The listing builds one solid part. Answer for the finished solid, in the listing's coordinates (mm). Round coordinates to 2 decimals unless told otherwise and drop trailing zeros. Order: outer loops, then holes, each group sorted by start corner. A loop starts at its lowest first (then second) coordinate and runs counter-clockwise, first axis right, second up. Notation, with made-up numbers: M 9,35.5 L 46,35.5 A21 cw 46,48.5 Z; hole C -11.75,-29 d5. An arc over 180 degrees is marked long. Put each result on its own line as item: value. Start each with the question number.
1. Consider line 1 (Y direction, x = 11.5, z = 546.1); line 2 (X direction, y = 8.25, z = 552). Determine where each line is inside the solid, lowest interval first.
2. The part is cut by section B-B (z = 322.5). Give the vertices of the cut face in (x, y), then the cut area to 3 significant figures.
3. The part is cut by section A-A (x = -5). Give the vertices of the cut face in (y, z), then the cut area to 3 significant figures.
Autodesk Inventor part; units mm, degrees
ref_plane "YZ Plane" through (0, 0, 0) normal (1, 0, 0) x (0, 1, 0)
ref_plane "XZ Plane" through (0, 0, 0) normal (0, 1, 0) x (-1, 0, 0)
ref_plane "XY Plane" through (0, 0, 0) normal (0, 0, 1) x (1, 0, 0)
sketch "Sketch1" plane through (0, 0, 0) normal (0, 0, 1) x (1, 0, 0)
  line L0 (-12.7, -12.7) -> (-12.7, 12.7)
  line L1 (-12.7, 12.7) -> (12.7, 12.7)
  line L2 (12.7, 12.7) -> (12.7, -12.7)
  line L3 (12.7, -12.7) -> (-12.7, -12.7)
  line L4 (-12.7, -12.7) -> (12.7, 12.7) construction
  line L5 (-12.7, 12.7) -> (12.7, -12.7) construction
  line L6 (11.1125, 11.1125) -> (-11.1125, 11.1125)
  line L7 (-11.1125, 11.1125) -> (-11.1125, -11.1125)
  line L8 (-11.1125, -11.1125) -> (11.1125, -11.1125)
  line L9 (11.1125, -11.1125) -> (11.1125, 11.1125)
  point P0 (0, 0)
  dimension "d0" = 25.4
  dimension "d1" = 25.4
  dimension "d2" = 1.5875
extrude "Extrusion1" add sketch "Sketch1" along normal blind 609.6
sketch "Sketch2" plane through (12.7, -12.7, 0) normal (1, 0, 0) x (0, 0, -1)
  line L0 (0, 0) -> (0, 25.4)
  line L1 (0, 25.4) -> (-609.6, 25.4)
  line L2 (-609.6, 0) -> (-609.6, 25.4)
  line L3 (0, 0) -> (-609.6, 0)
  circle A0 centre (-596.9, 12.7) radius 2.5781
  circle A1 centre (-571.5, 12.7) radius 2.5781
  circle A2 centre (-546.1, 12.7) radius 2.5781
  line L4 (-304.8, 0) -> (-304.8, 25.4) construction
  circle A3 centre (-12.7, 12.7) radius 2.5781
  circle A4 centre (-38.1, 12.7) radius 2.5781
  circle A5 centre (-63.5, 12.7) radius 2.5781
  point P0 (0, 12.7)
  dimension "d5" = 5.1562
  dimension "d7" = 12.7
  dimension "d8" = 25.4
  dimension "d9" = 25.4
extrude "Extrusion2" cut sketch "Sketch2" against normal through all contours A0 | A1 | A2 | A3 | A4 | A5
equation "\"d1\" = d0"
properties part number "24in long 1in square tube"
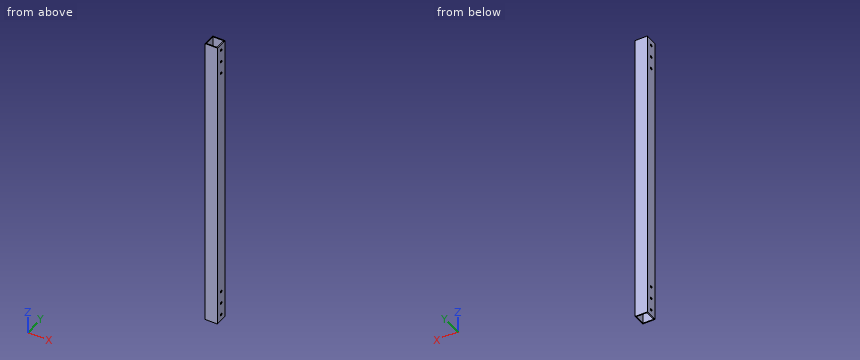
Resolved:
1. line 1: -12.7 to -2.58, 2.58 to 12.7
1. line 2: -12.7 to -11.11, 11.11 to 12.7
2. outline: M -12.7,-12.7 L 12.7,-12.7 L 12.7,12.7 L -12.7,12.7 Z; hole M -11.11,-11.11 L 11.11,-11.11 L 11.11,11.11 L -11.11,11.11 Z
2. area: 151 mm2
3. outline: M -12.7,0 L -11.11,0 L -11.11,609.6 L -12.7,609.6 Z; M 11.11,0 L 12.7,0 L 12.7,609.6 L 11.11,609.6 Z
3. area: 1,940 mm2
